Autodesk Inventor part; units mm, degrees
ref_plane "YZ Plane" through (0, 0, 0) normal (1, 0, 0) x (0, 1, 0)
ref_plane "XZ Plane" through (0, 0, 0) normal (0, 1, 0) x (-1, 0, 0)
ref_plane "XY Plane" through (0, 0, 0) normal (0, 0, 1) x (1, 0, 0)
sketch "Skizze1" plane through (0, 0, 0) normal (0, 0, 1) x (1, 0, 0)
  arc A0 (-1.5, 4.7697) -> (1.5, 4.7697) centre (0, 0) ccw
  circle A1 centre (0, 0) radius 13
  line L0 (-33.9343, 0) -> (76.2277, 0) construction
  circle A2 centre (0, 0) radius 17.5
  circle A3 centre (45, 112.9423) radius 15
  line L1 (60, 112.9423) -> (60, 192.9423)
  line L2 (30, 112.9423) -> (30, 192.9423)
  line L3 (45, 112.9423) -> (45, 207.9423) construction
  line L4 (45, 112.9423) -> (45, 127.9423) construction
  line L5 (30, 112.9423) -> (60, 112.9423) construction
  line L6 (-17.5, 0) -> (-17.5, 35)
  line L7 (17.5, 0) -> (17.5, 35)
  line L8 (-17.5, 35) -> (17.5, 35) construction
  circle A4 centre (0, 35) radius 17.5 construction
  line L9 (-14.6522, 44.5688) -> (30, 112.9423)
  arc A5 (-14.6522, 44.5688) -> (-17.5, 35) centre (0, 35) ccw
  line L10 (17.5, 35) -> (58.0047, 105.4671)
  arc A6 (58.0047, 105.4671) -> (60, 112.9423) centre (45, 112.9423) ccw
  line L11 (0, 35) -> (45, 112.9423) construction
  circle A7 centre (45, 192.9423) radius 15
  circle A8 centre (45, 192.9423) radius 5
  circle A9 centre (45, 112.9423) radius 5
  line L12 (-1.5, 6.4) -> (1.5, 6.4)
  line L13 (1.5, 6.4) -> (1.5, 4.7697)
  line L14 (-1.5, 4.7697) -> (-1.5, 6.4)
  line L15 (0, 0) -> (0, 5) construction
  line L16 (0, 5) -> (1.5, 5) construction
  point P0 (22.5, 73.9711)
  point P1 (45, 152.9423)
  point P2 (-13, 0)
  point P3 (13, 0)
  point P4 (0, 6.4)
  dimension "d0" = 10
  dimension "d1" = 26
  dimension "d4" = 35
  dimension "d36" = 0
  dimension "d37" = 30
  dimension "d38" = 60
  dimension "d39" = 35
  dimension "d40" = 90
  dimension "d41" = 80
  dimension "d42" = 45
  dimension "d43" = 10
  dimension "d44" = 10
  dimension "d45" = 40
  dimension "d51" = 3
  dimension "d52" = 1.4
extrude "Extrusion1" add sketch "Skizze1" against normal blind 5 contours A1 | A3 | A7
extrude "Extrusion2" add sketch "Skizze1" along normal blind 8 contours A1 | A2 | A2 L6 A5 L9 A3 L10 L7 | A3 | L2 A7 L1 A3 | A7
fillet "Rundung1" radius 25 2 edges at (30, 112.9423, 4) (17.5, 35, 4)
hole "Bohrung2" at (45, 152.9423, 0) at (22.5, 73.9711, 0) direction (0, 0, 1) diameter 8 end through all
ref_plane "Arbeitsebene1" through (45, 112.9423, 0) normal (1, 0, 0) x (0, 0, -1)
sketch "Skizze3" plane through (45, 112.9423, 0) normal (1, 0, 0) x (0, 0, -1)
  line L0 (-10.6, 0) -> (7.6, 0) construction
  line L1 (-10.6, 80) -> (7.6, 80) construction
  line L2 (-8, 91) -> (-2, 91)
  line L3 (-2, 91) -> (-2, 90)
  line L4 (-2, 90) -> (-1.5, 90)
  line L5 (-1.5, 90) -> (-1.5, 87.5)
  line L6 (-1.5, 87.5) -> (2, 87.5)
  line L7 (-8, 75) -> (-8, 85) construction
  line L8 (5, 85) -> (-8, 85) construction
  line L9 (5, 75) -> (-8, 75) construction
  line L10 (5, 85) -> (5, 75) construction
  line L11 (0, 0) -> (0, 80) construction
  line L12 (2, 87.5) -> (2, 92)
  line L13 (2, 92) -> (5, 92)
  line L14 (-8, 91) -> (-8, 85)
  line L15 (5, 92) -> (5, 85)
  line L16 (-8, 85) -> (5, 85)
  point P0 (0, -112.9423)
  dimension "d53" = 6
  dimension "d54" = 22
  dimension "d55" = 20
  dimension "d56" = 15
  dimension "d57" = 24
  dimension "d58" = 3
  dimension "d59" = 0.5
revolve "Umdrehung1" cut sketch "Skizze3" angle 360 about axis through (45, 192.9423, 0) along (0, 0, -1)
pattern_linear "Rechteckige Anordnung1" count 2 spacing 80 along (0, -1, 0) of "Umdrehung1"
properties part number "ParallelSystem_ProximalPart_Driven_v2" material "Edelstahl"
Can you work these out from the model? Positions are in its coordinate system, mm. A direction names the side the tool comes from. Give positions to 0.01 mm unless a question says otherwise; leave off trailing zeros. Order: outer loops, then holes, each group sorted by start corner. A loop starts at its lowest first (then second) coordinate and runs counter-clockwise, first axis right, second up. Notation, with made-up numbers: M 61.25,40.5 L 100.25,40.5 A18 ccw 100.25,53.5 Z; hole C -15.75,4.25 d11. An arc over 180 degrees is marked long. One line per item, written item: value.
1) For P1, Ø18, axis at x = 45, y = 192.94, coming from the +Z side; P2, Ø2, axis at x = 0.5, z = -0.5, coming from the -Y side; P3, Ø4, axis at x = 7, z = 5.5, coming from the -Y side; P4, Ø2, axis at x = 18, y = 6, coming from the -Z side, each with a flat end and sliding along its axis, tell me the tip position at first contact or that it passes through.
Answer sheet:
P1: stops at z = 1.5
P2: stops at y = -17.5
P3: stops at y = -16.77
P4: stops at z = 0
2) On a 3-axis mill with a long thin cutter (end or side, diameter ignored), from which of +Z, -Z, +X, -X, +Y, -Y can I reach the whole of each face in a straight line? I mean faces 1 (the face through (36.13, 117.56, 1.75)), 2 (the face through (18.37, 34.86, 4.06)), 3 (the face through (48.6, 204.39, -3.52)). Say none if no direction works.
Answer sheet:
face 1: +Z
face 2: +Z, -Z, +X, -Y
face 3: -Z
3) I want a section at B-B, the plane y = 115. List the corners of the cut face in (x, z) for me, plus the area to 3 significant figures.
Answer sheet:
outline: M 29.41,0 L 30.14,0 L 30.14,-5 L 33.18,-5 L 33.18,-2 L 37.79,-2 L 37.79,1.5 L 35.21,1.5 L 35.21,2 L 34.19,2 L 34.19,8 L 29.41,8 Z; M 52.21,-2 L 56.82,-2 L 56.82,-5 L 59.86,-5 L 59.86,0 L 60,0 L 60,8 L 55.81,8 L 55.81,2 L 54.79,2 L 54.79,1.5 L 52.21,1.5 Z
area: 132 mm^2
4) I want a section at A-A, the plane z = 5. List the corners of the cut face in (x, y) for me, plus the area to 3 significant figures.
Answer sheet:
outline: M -17.5,0 A17.5 ccw 17.5,0 L 17.5,28.33 A25 cw 20.83,40.79 L 58,105.47 A15 ccw 60,112.94 L 60,192.94 A15 ccw 30,192.94 L 30,120.38 A25 cw 25.93,106.71 L -14.65,44.57 A17.5 ccw -17.5,35 Z; hole M -1.5,4.77 A5 ccw long 1.5,4.77 L 1.5,6.4 L -1.5,6.4 Z; hole C 22.5,73.97 d8; hole C 45,112.94 d22; hole C 45,192.94 d22; hole C 45,152.94 d8
area: 6,260 mm^2
5) I want a section at C-C, the plane x = 45. Count the separate pieces of the cut face and the enclosed holes in it, plus the area to 3 significant figures.
Answer sheet:
separate pieces: 4
enclosed holes: 0
area: 704 mm^2
6) I want a section at D-D, the plane y = 138.5. List the corners of the cut face in (x, z) for me.
Answer sheet:
outline: M 30,0 L 60,0 L 60,8 L 30,8 Z
7) Please list where these lines run through material, in increasing order: line 1 along Y through (x, z) = (45.5, -1.25); line 2 along Z through (x, y) = (-6, 42.5); line 3 along Y through (x, z) = (22.5, 2.25).
Answer sheet:
line 1: y = 97.95 to 105.46, 120.43 to 127.93, 177.95 to 185.46, 200.43 to 207.93
line 2: z = 0 to 8
line 3: y = 43.7 to 69.97, 77.97 to 101.46
